Verification items for the finished model (mm, model axes). Round coordinates to 2 decimals unless told otherwise and drop trailing zeros. Loops run counter-clockwise (first coordinate to the right, second up) from the corner with the lowest first, then second, coordinate; pieces in that order, holes last. Notation, with made-up numbers: (25.25, -34) -> (32.25, -34) arc R19 cw to (32.25, -3) -> close; hole circle Ø9 at (10.5, -29.5). An arc over 180 degrees is marked (long way). Write item = value, one per line.
Autodesk Inventor part; units mm, degrees
ref_plane "YZ Plane" through (0, 0, 0) normal (1, 0, 0) x (0, 1, 0)
ref_plane "XZ Plane" through (0, 0, 0) normal (0, 1, 0) x (-1, 0, 0)
ref_plane "XY Plane" through (0, 0, 0) normal (0, 0, 1) x (1, 0, 0)
sketch "Sketch1" plane through (0, 0, 0) normal (0, 1, 0) x (-1, 0, 0)
  line L0 (10.9985, -6.35) -> (0, -12.7)
  line L1 (0, -12.7) -> (-10.9985, -6.35)
  line L2 (-10.9985, -6.35) -> (-10.9985, 6.35)
  line L3 (-10.9985, 6.35) -> (0, 12.7)
  line L4 (0, 12.7) -> (10.9985, 6.35)
  line L5 (10.9985, 6.35) -> (10.9985, -6.35)
  point P0 (0, 0)
  point P1 (0, 0)
  dimension "d2" = 25.4
extrude "Extrusion1" add sketch "Sketch1" along normal blind 12.7
sketch "Sketch2" plane through (0, 12.7, 0) normal (0, 1, 0) x (1, 0, 0)
  circle A0 centre (0, 0) radius 10.9985
extrude "Extrusion2" cut sketch "Sketch2" against normal through all draft 45 keep common part
sketch "Sketch3" plane through (0, 0, 0) normal (0, -1, 0) x (1, 0, 0)
  circle A0 centre (0, 0) radius 10.9985
extrude "Extrusion3" cut sketch "Sketch3" against normal through all draft 45 keep common part
sketch "Sketch4" plane through (0, 0, 0) normal (0, -1, 0) x (1, 0, 0)
  circle A0 centre (0, 0) radius 5.08
  dimension "d9" = 10.16
extrude "Extrusion4" cut sketch "Sketch4" against normal through all
properties part number "Nut"
(1) Material ranges on probe 1 along X at (y, z) = (10.75, 1); probe 2 along X at (y, z) = (10.25, 3.25); probe 3 along Z at (x, y) = (0.5, 8), recorded low to high. Write a range as from..to.
Filled sheet:
probe_1 = -11..-4.98, 4.98..11
probe_2 = -11..-3.9, 3.9..11
probe_3 = -12.41..-5.06, 5.06..12.41
(2) Go/stop test with flat-tipped pins: pin 1 Ø3 at (x, y) = (6, 7.5) entering from -Z; pin 2 Ø3 at (x, y) = (-4, 6.5) entering from +Z; pin 3 Ø1 at (x, y) = (7, 2.5) entering from +Z. Record where each tip stops, or that it passes through.
Filled sheet:
pin_1 = -10.1
pin_2 = 11.26
pin_3 = 8.95
(3) Sectioned sample at A-A, the plane y = 10.25. Record the cut outline in (x, z).
Filled sheet:
outline = (-11, -6.35) -> (0, -12.7) -> (11, -6.35) -> (11, 6.35) -> (0, 12.7) -> (-11, 6.35) -> close; hole circle Ø10.16 at (0, 0)
